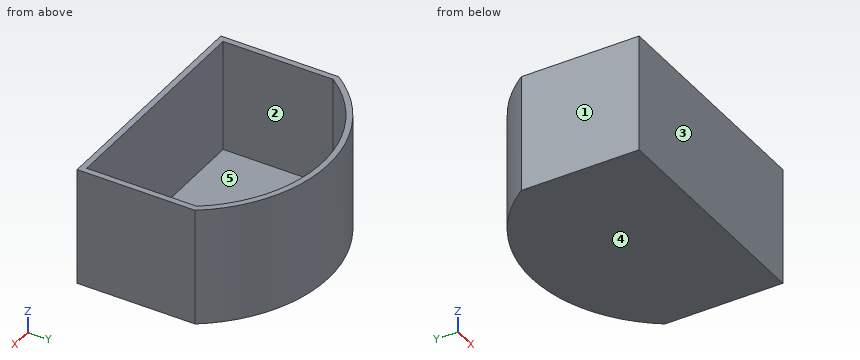
from build123d import *

# Parameters (mm, degrees)
F1_DEPTH = 50.8
F2_T     = -2.54


with BuildPart() as f1:
    # F0 (on Top) → F1 (new body)
    with BuildSketch(Plane.XY):
        with BuildLine():
            Line((-50.8, 25.4), (-50.8, -25.4))
            Line((-50.8, -25.4), (50.8, -25.4))
            Line((50.8, -25.4), (50.8, 25.4))
            ThreePointArc((50.8, 25.4), (0, 51.874105), (-50.8, 25.4))
        make_face()
    extrude(amount=F1_DEPTH)

    # F2
    f2_openings = [f1.faces().sort_by_distance(p)[0] for p in [
        (0, 9.695027, 50.8),
    ]]
    offset(amount=F2_T, openings=f2_openings)


solid = f1.part
Here's how the part is built. I have some questions about the finished solid (model axes, mm). Face numbers are marked on the shaded views. A direction names the side the tool comes from. Round coordinates to 2 decimals unless told otherwise and drop trailing zeros. Write each loop counter-clockwise with the first axis right and the second up, starting at its lowest first coordinate (ties: lowest second). Pieces come first, ordered by that corner, then holes.
1. Suppose I cut it at C-C (x = 30.5). List the corners of the cut face in (y, z) for me.
2. Suppose I cut it at A-A (z = 23). List the corners of the cut face in (x, y) for me.
3. Will these pins go through, and if not, where does the flat tip stop? pin 1 Ø10 at (x, y) = (-1.5, 4) entering from +Z; pin 2 Ø4 at (x, z) = (-15, 11) entering from +Y; pin 3 Ø12 at (x, z) = (-4.5, 24.5) entering from +Y.
4. Suppose I cut it at B-B (y = -2). List the corners of the cut face in (x, z) for me.
5. I need wall thicknesses on L1, parallel to X at y = 11, z = 36; L2, parallel to Z at x = -25, y = 37.5; L3, parallel to Y at x = -18, z = 23.5. Which ranges of each line are inside material? Lowest first, please.
6. For the marked faces 4 and 5, which set-ups out of +Z, -Z, +X, -X, +Y, -Y let a thin tool reach every point of the face, with its end or its side?
7. If we mould it in two halves opening along Y, with no side actions, what happens to the marked faces 1, 2 and 3? For each: released by +Y, released by -Y, zero draft, split by the parting line, or undercut.
Answer sheet:
1. outline: (-25.4, 0) - (43.85, 0) - (43.85, 50.8) - (40.91, 50.8) - (40.91, 2.54) - (-22.86, 2.54) - (-22.86, 50.8) - (-25.4, 50.8) - close
2. outline: (-50.8, -25.4) - (50.8, -25.4) - (50.8, 25.4) arc R61.98 ccw to (-50.8, 25.4) - close; hole (-48.26, -22.86) - (48.26, -22.86) - (48.26, 24.59) arc R59.44 ccw to (-48.26, 24.59) - close
3. pin 1: stops at z = 2.54
3. pin 2: stops at y = 50.5
3. pin 3: stops at y = 51.87
4. outline: (-50.8, 0) - (50.8, 0) - (50.8, 50.8) - (48.26, 50.8) - (48.26, 2.54) - (-48.26, 2.54) - (-48.26, 50.8) - (-50.8, 50.8) - close
5. L1: x = -50.8 to -48.26, 48.26 to 50.8
5. L2: z = 0 to 2.54
5. L3: y = -25.4 to -22.86, 46.54 to 49.2
6. face 4: -Z, +X, -X, +Y, -Y
6. face 5: +Z
7. face 1: zero draft
7. face 2: undercut
7. face 3: released by -Y
